Autodesk Inventor part; units mm, degrees
ref_plane "YZ Plane" through (0, 0, 0) normal (1, 0, 0) x (0, 1, 0)
ref_plane "XZ Plane" through (0, 0, 0) normal (0, 1, 0) x (-1, 0, 0)
ref_plane "XY Plane" through (0, 0, 0) normal (0, 0, 1) x (1, 0, 0)
sketch "Sketch1" plane through (0, 0, 0) normal (0, 1, 0) x (-1, 0, 0)
  line L0 (-70.0685, 0) -> (70.0685, 0) construction
  line L1 (0, -20.6438) -> (0, 20.6438) construction
  line L2 (65, -55) -> (-65, -55)
  line L3 (-65, -55) -> (-65, 55)
  line L4 (-65, 55) -> (65, 55)
  line L5 (65, 55) -> (65, -55)
  point P0 (0, 0)
  point P1 (0, 0)
  dimension "d0" = 110
  dimension "d1" = 130
extrude "Extrusion1" add sketch "Sketch1" along normal blind 5
sketch "Sketch2" plane through (0, 0, 0) normal (0, -1, 0) x (1, 0, 0)
  line L0 (-160.533, 0) -> (160.533, 0) construction
  line L1 (0, 8.6003) -> (0, -8.6003) construction
  line L2 (-57.5, 45) -> (-52.5, 45) construction
  line L3 (-57.5, 47.5) -> (-52.5, 47.5)
  line L4 (-52.5, 42.5) -> (-57.5, 42.5)
  arc A0 (-57.5, 47.5) -> (-57.5, 42.5) centre (-57.5, 45) ccw
  arc A1 (-52.5, 42.5) -> (-52.5, 47.5) centre (-52.5, 45) ccw
  line L5 (57.5, 45) -> (52.5, 45) construction
  line L6 (57.5, 47.5) -> (52.5, 47.5)
  line L7 (52.5, 42.5) -> (57.5, 42.5)
  arc A2 (57.5, 42.5) -> (57.5, 47.5) centre (57.5, 45) ccw
  arc A3 (52.5, 47.5) -> (52.5, 42.5) centre (52.5, 45) ccw
  line L8 (57.5, -45) -> (52.5, -45) construction
  line L9 (57.5, -42.5) -> (52.5, -42.5)
  line L10 (52.5, -47.5) -> (57.5, -47.5)
  arc A4 (57.5, -47.5) -> (57.5, -42.5) centre (57.5, -45) ccw
  arc A5 (52.5, -42.5) -> (52.5, -47.5) centre (52.5, -45) ccw
  line L11 (-57.5, -45) -> (-52.5, -45) construction
  line L12 (-57.5, -47.5) -> (-52.5, -47.5)
  line L13 (-52.5, -42.5) -> (-57.5, -42.5)
  arc A6 (-57.5, -42.5) -> (-57.5, -47.5) centre (-57.5, -45) ccw
  arc A7 (-52.5, -47.5) -> (-52.5, -42.5) centre (-52.5, -45) ccw
  point P0 (0, 0)
  point P1 (-55, 45)
  point P2 (55, 45)
  point P3 (55, -45)
  point P4 (-55, -45)
  point P5 (0, 0)
  point P6 (-60, 45)
  point P7 (-50, 45)
  dimension "d4" = 110
  dimension "d5" = 90
  dimension "d7" = 5
  dimension "d8" = 10
extrude "Extrusion2" cut sketch "Sketch2" against normal through all
sketch "Sketch3" plane through (0, 0, 0) normal (0, -1, 0) x (1, 0, 0)
  line L0 (-38.6076, 0) -> (38.6076, 0) construction
  line L1 (0, -3.4177) -> (0, 3.4177) construction
  line L2 (10, -10) -> (-10, -10)
  line L3 (-10, -10) -> (-10, 10)
  line L4 (-10, 10) -> (10, 10)
  line L5 (10, 10) -> (10, -10)
  point P0 (0, 0)
  point P1 (0, 0)
  dimension "d11" = 20
  dimension "d12" = 20
extrude "Extrusion3" add sketch "Sketch3" against normal blind 75
sketch "Sketch4" plane through (-10, 5, 10) normal (0, 0, 1) x (1, 0, 0)
  line L0 (20, 70) -> (0, 70)
  circle A0 centre (10, 70) radius 65
  point P0 (10, -5)
  dimension "d15" = 130
extrude "Extrusion4" add sketch "Sketch4" along normal up to surface (45 mm away)
sketch "Sketch5" plane through (0, 75, 55) normal (0, 0, 1) x (1, 0, 0)
  line L0 (10, 0) -> (-10, 0)
  circle A0 centre (0, 0) radius 35
  point P0 (0, -75)
  dimension "d18" = 70
extrude "Extrusion5" add sketch "Sketch5" along normal blind 55
sketch "Sketch6" plane through (0, 75, 110) normal (0, 0, 1) x (1, 0, 0)
  arc A0 (-2, 5.6569) -> (2, 5.6569) centre (0, 0) ccw
  circle A1 centre (0, 0) radius 35
  line L0 (-2, 7.6569) -> (2, 7.6569)
  line L1 (2, 7.6569) -> (2, 5.6569)
  line L2 (-2, 5.6569) -> (-2, 7.6569)
  point P0 (0, -75)
  dimension "d21" = 12
  dimension "d23" = 2
  dimension "d26" = 4
  dimension "d27" = 2
extrude "Extrusion6" add sketch "Sketch6" along normal blind 15 contours L2 L0 L1 A0
sketch "Sketch8" plane through (-10, 5, 10) normal (0, 0, -1) x (-1, 0, 0)
  arc A0 (-12, 75.6569) -> (-8, 75.6569) centre (-10, 70) ccw
  circle A1 centre (-10, 70) radius 65
  arc A2 (0, 5.7738) -> (-20, 5.7738) centre (-10, 70) ccw
  point P0 (-10, -5)
extrude "Extrusion7" add sketch "Sketch8" along normal blind 135
properties part number "MotorV1"
Model file for the job. Use its own axes, mm. A direction names the side the tool comes from. Coordinates: 2 decimals unless noted, no trailing zeros. Loops run counter-clockwise (first coordinate to the right, second up) from the corner with the lowest first, then second, coordinate; pieces in that order, holes last. Notation, with made-up numbers: (5, 1) - (14, 1) arc R26 ccw to (14, 35) - close; hole circle Ø7 at (24, 53). An arc over 180 degrees is marked (long way). Write item = value, one per line. Start each with the question number.
Item 1: Drop flat-ended pins along their axis: pin 1 Ø5.5 at (x, y) = (-15, 2.5) entering from +Z; pin 2 Ø8 at (x, y) = (-29.5, 61) entering from +Z; pin 3 Ø5.5 at (x, y) = (-56, 1.5) entering from -Z. Give the stop position or say it passes through.
Item 2: Saw through at A-A, the plane z = -17.5. List the corners of the cut face in (x, y).
Item 3: Saw through at D-D, the plane x = 39.5. List the corners of the cut face in (y, z), then the cut area to 3 significant figures.
Item 4: Saw through at B-B, the plane x = -43.5. List the corners of the cut face in (y, z).
Item 5: Pull direction X, two halves, no side cores. Call faces 1 (the face through (-65, 2, 1)), 2 (the face through (-1, 2, -55)), 3 (the face through (55, 2, -47.5)): +X half, -X half, draft (parallel to the pull), parting line (faces both ways), or undercut.
Item 6: Saw through at C-C, the plane y = 75. List the corners of the cut face in (x, z), then the cut area to 3 significant figures.
Item 7: Wall check: probe 1 along Y at (x, z) = (0.5, 48); probe 2 along Z at (x, y) = (13.5, 48.5); probe 3 along Z at (x, y) = (-18, 31). Give the ranges that are in metal, low to high. Write a range as [from, to].
Item 8: 3-axis set-ups, long thin cutter, end or side, ignore diameter. For faces 4 (the face through (-4.56, 40.3, 82.12)), 5 (the face through (1, 2, 55)), 6 (the face through (0, 76, 125)), 7 (the face through (-55, 2, 47.5)): which of +Z, -Z, +X, -X, +Y, -Y reach the whole face in a straight line?
Answers:
q1.pin_1 = 55
q1.pin_2 = 110
q1.pin_3 = -55
q2.outline = (-65, 0) - (65, 0) - (65, 5) - (-65, 5) - close; circle Ø130 at (0, 75)
q3.outline = (0, -55) - (5, -55) - (5, 55) - (0, 55) - close; (23.38, -125) - (126.62, -125) - (126.62, 55) - (23.38, 55) - close
q3.area = 19,100 mm2
q4.outline = (0, -55) - (5, -55) - (5, 55) - (0, 55) - close; (26.7, -125) - (123.3, -125) - (123.3, 55) - (26.7, 55) - close
q5.face_1 = -X half
q5.face_2 = draft
q5.face_3 = undercut
q6.outline = (-65, -125) - (65, -125) - (65, 55) - (35, 55) - (35, 110) - (6, 110) - (6, 125) - (-6, 125) - (-6, 110) - (-35, 110) - (-35, 55) - (-65, 55) - close
q6.area = 27,400 mm2
q7.probe_1 = [0, 5], [10, 140]
q7.probe_2 = [-125, 110]
q7.probe_3 = [-125, 55]
q8.face_4 = +Z
q8.face_5 = +Z, +X, -X, -Y
q8.face_6 = +Z, +X, -X, +Y, -Y
q8.face_7 = -Y
